The model under review builds one solid part; all positions refer to its coordinate system, in mm. Round coordinates to 2 decimals unless told otherwise and drop trailing zeros. Order: outer loops, then holes, each group sorted by start corner. A loop starts at its lowest first (then second) coordinate and runs counter-clockwise, first axis right, second up. Notation, with made-up numbers: M 27.5,-28.5 L 43.5,-28.5 A8 ccw 43.5,-20.5 Z; hole C -15.75,-3 d7. An arc over 180 degrees is marked long. One line per item, written item: value. Start each with the question number.
from build123d import *

# Parameters (mm, degrees)
SKETCH_1_W                   = 80
SKETCH_1_H                   = 50
EXTRUDE_1_DEPTH              = 3
EXTRUDE_2_DEPTH              = 3
SKETCH_8_R                   = 1.5
CUT_EXTRUDE_4_DEPTH          = 3
CUT_EXTRUDE_START            = -4
CUT_EXTRUDE_6_DEPTH          = 5
HOLE_WIZARD_M3_1_D           = 3
HOLE_WIZARD_M3_1_CSINK_D     = 6
HOLE_WIZARD_M3_1_CSINK_ANGLE = 90
MIRROR_7_COPY_1_DEPTH        = 3
MIRROR_START                 = -4
MIRROR_7_COPY_2_DEPTH        = 5
MIRROR_7_COPY_3_D            = 3
MIRROR_7_COPY_3_CSINK_D      = 6
MIRROR_7_COPY_3_CSINK_ANGLE  = 90
SKETCH_14_R                  = 10.1
CUT_EXTRUDE_7_DEPTH          = 4
SKETCH_15_R                  = 1.5
CUT_EXTRUDE_8_DEPTH          = 10
MIRROR_9_COPY_1_SKETCH_R     = 1.5
MIRROR_9_COPY_1_DEPTH        = 10


with BuildPart() as part:
    # 草图1 → 凸台-拉伸1 (new body)
    with BuildSketch(Plane(origin=(0, 0, 0), x_dir=(1, 0, 0), z_dir=(0, 1, 0))):
        Polygon((-15, -105.5), (-40, -25), (40, -25), (15, -105.5), align=None)
        Rectangle(SKETCH_1_W, SKETCH_1_H)
        Polygon((-15, 105.5), (15, 105.5), (40, 25), (-40, 25), align=None)
    extrude(amount=EXTRUDE_1_DEPTH)

    # 草图7 → 凸台-拉伸2 (add)
    with BuildSketch(Plane(origin=(0, 3, 0), x_dir=(1, 0, 0), z_dir=(0, 1, 0))):
        Polygon((15, 105.5), (25.392304845, 111.5), (31.392304845, 111.5), (34.279056191, 106.5), (31.392304845, 101.5), (27.5, 65.25), align=None)
    extrude_2 = extrude(amount=-EXTRUDE_2_DEPTH)

    # 草图8 → 切除-拉伸4 (cut)
    with BuildSketch(Plane(origin=(0, 3, 0), x_dir=(1, 0, 0), z_dir=(0, 1, 0))):
        with Locations((27, 106.5)):
            Circle(SKETCH_8_R)
    extrude(amount=-CUT_EXTRUDE_4_DEPTH, mode=Mode.SUBTRACT)

    # 草图9 → 切除-拉伸6 (cut)
    with BuildSketch(Plane(origin=(0, 3, 0), x_dir=(1, 0, 0), z_dir=(0, 1, 0)).offset(CUT_EXTRUDE_START)):
        Polygon((22.528576043, 65.783801312), (26.420880888, 102.033801312), (23.243297221, 103.222190391), (21.66924243, 105.948533263), (16.658152368, 102.627995852), (19.093364206, 84.205898582), (21.528576043, 65.783801312), align=None)
        Polygon((10.313400805, 97.671116845), (19.093364206, 84.205898582), (16.658152368, 102.627995852), (9.970725358, 98.196654308), align=None)
    cut_extrude_6 = extrude(amount=CUT_EXTRUDE_6_DEPTH, mode=Mode.SUBTRACT)

    # M3 六角凹锥坑螺钉的锥形沉头孔1 (through all)
    with Locations(Plane(origin=(0, 3, 0), x_dir=(1, 0, 0), z_dir=(0, 1, 0))):
        with Locations((27, 106.5), (32, 0)):
            hole_wizard_m3_1 = CounterSinkHole(HOLE_WIZARD_M3_1_D / 2, HOLE_WIZARD_M3_1_CSINK_D / 2, counter_sink_angle=HOLE_WIZARD_M3_1_CSINK_ANGLE)

    # 镜向5: M3 六角凹锥坑螺钉的锥形沉头孔1 across plane
    add(hole_wizard_m3_1.mirror(Plane(origin=(0, 0, 0), x_dir=(0, 0, 1), z_dir=(1, 0, 0))), mode=Mode.SUBTRACT)

    # 镜向6: 凸台-拉伸2, 切除-拉伸6, M3 六角凹锥坑螺钉的锥形沉头孔1 across plane
    add(extrude_2.mirror(Plane(origin=(0, 0, 0), x_dir=(0, 0, 1), z_dir=(1, 0, 0))))
    add(cut_extrude_6.mirror(Plane(origin=(0, 0, 0), x_dir=(0, 0, 1), z_dir=(1, 0, 0))), mode=Mode.SUBTRACT)
    add(hole_wizard_m3_1.mirror(Plane(origin=(0, 0, 0), x_dir=(0, 0, 1), z_dir=(1, 0, 0))), mode=Mode.SUBTRACT)

    # 镜向7: 凸台-拉伸2, 切除-拉伸6, M3 六角凹锥坑螺钉的锥形沉头孔1 across plane
    add(extrude_2.mirror(Plane.XY))
    add(cut_extrude_6.mirror(Plane.XY), mode=Mode.SUBTRACT)
    add(hole_wizard_m3_1.mirror(Plane.XY), mode=Mode.SUBTRACT)

    # 镜向7 copy 1 sketch → 镜向7 copy 1 (add)
    with BuildSketch(Plane(origin=(0, 3, 0), x_dir=(-1, 0, 0), z_dir=(0, 1, 0))):
        Polygon((15, 105.5), (25.392304845, 111.5), (31.392304845, 111.5), (34.279056191, 106.5), (31.392304845, 101.5), (27.5, 65.25), align=None)
    extrude(amount=-MIRROR_7_COPY_1_DEPTH)

    # 镜向7 copy 2 sketch → 镜向7 copy 2 (cut)
    with BuildSketch(Plane(origin=(0, 3, 0), x_dir=(-1, 0, 0), z_dir=(0, 1, 0)).offset(MIRROR_START)):
        Polygon((22.528576043, 65.783801312), (26.420880888, 102.033801312), (23.243297221, 103.222190391), (21.66924243, 105.948533263), (16.658152368, 102.627995852), (19.093364206, 84.205898582), (21.528576043, 65.783801312), align=None)
        Polygon((10.313400805, 97.671116845), (19.093364206, 84.205898582), (16.658152368, 102.627995852), (9.970725358, 98.196654308), align=None)
    extrude(amount=MIRROR_7_COPY_2_DEPTH, mode=Mode.SUBTRACT)

    # 镜向7 copy 3 (through all)
    with Locations(Plane(origin=(0, 3, 0), x_dir=(-1, 0, 0), z_dir=(0, 1, 0))):
        with Locations((27, 106.5), (32, 0)):
            CounterSinkHole(MIRROR_7_COPY_3_D / 2, MIRROR_7_COPY_3_CSINK_D / 2, counter_sink_angle=MIRROR_7_COPY_3_CSINK_ANGLE)

    # 草图14 → 切除-拉伸7 (cut, through all)
    with BuildSketch(Plane(origin=(0, 3, 0), x_dir=(1, 0, 0), z_dir=(0, 1, 0))):
        Circle(SKETCH_14_R)
        with Locations((0, -50)):
            Circle(SKETCH_14_R)
        with Locations((0, 50)):
            Circle(SKETCH_14_R)
    extrude(amount=-CUT_EXTRUDE_7_DEPTH, mode=Mode.SUBTRACT)

    # 草图15 → 切除-拉伸8 (cut)
    with BuildSketch(Plane.XZ):
        with Locations((-32, 15)):
            Circle(SKETCH_15_R)
        with Locations((-32, 30)):
            Circle(SKETCH_15_R)
        with Locations((-12, 65)):
            Circle(SKETCH_15_R)
        with Locations((-12, 30)):
            Circle(SKETCH_15_R)
    cut_extrude_8 = extrude(amount=-CUT_EXTRUDE_8_DEPTH, mode=Mode.SUBTRACT)

    # 镜向8: 切除-拉伸8 across plane
    add(cut_extrude_8.mirror(Plane(origin=(0, 0, 0), x_dir=(0, 0, 1), z_dir=(1, 0, 0))), mode=Mode.SUBTRACT)

    # 镜向9: 切除-拉伸8 across plane
    add(cut_extrude_8.mirror(Plane.XY), mode=Mode.SUBTRACT)

    # 镜向9 copy 1 sketch → 镜向9 copy 1 (cut)
    with BuildSketch(Plane(origin=(0, 0, 0), x_dir=(-1, 0, 0), z_dir=(0, -1, 0))):
        with Locations((-32, 15)):
            Circle(MIRROR_9_COPY_1_SKETCH_R)
        with Locations((-32, 30)):
            Circle(MIRROR_9_COPY_1_SKETCH_R)
        with Locations((-12, 65)):
            Circle(MIRROR_9_COPY_1_SKETCH_R)
        with Locations((-12, 30)):
            Circle(MIRROR_9_COPY_1_SKETCH_R)
    extrude(amount=-MIRROR_9_COPY_1_DEPTH, mode=Mode.SUBTRACT)


solid = part.part
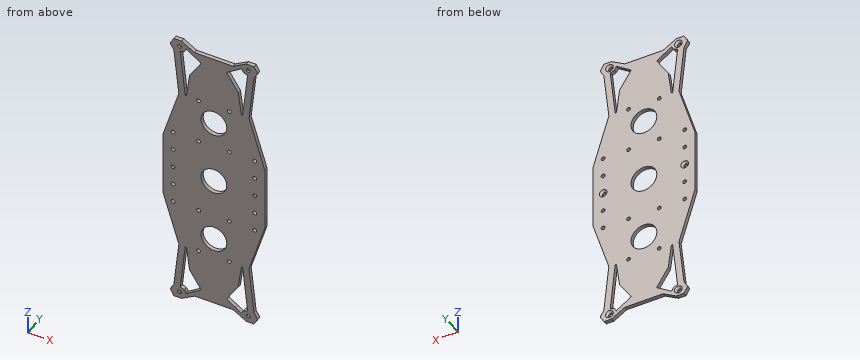
Item 1: Clearance check with flat-ended pins moving along their axes: P1, Ø1, axis at y = 1.5, z = 72.5, coming from the -X side; P2, Ø12, axis at x = 0, z = -50, coming from the +Y side; P3, Ø1.5, axis at x = 3, y = 1.5, coming from the +Z side; P4, Ø5, axis at x = 27, z = 106.5, coming from the +Y side. State where each tip first meets the part, or that it passes through.
Item 2: Consider section B-B, the plane y = 2.35. Count the separate pieces of the cut face and the enclosed holes in it, then the cut area to 3 significant figures.
Item 3: Consider section C-C, the plane z = 50. Give the boundary of the cut face in (x, y), then the cut area to 3 significant figures.
Item 4: Consider section A-A, the plane z = 87. Give the boundary of the cut face in (x, y), then the cut area to 3 significant figures.
Item 5: Wall thickness on L1, parallel to Z at x = 0, y = 2.35; L2, parallel to X at y = 0.8, z = -106.5; L3, parallel to X at y = 1.7, z = -14.5: over which ranges is each line inside the solid? List them lowest first.
Item 6: Consider section D-D, the plane z = -93.5. Give the boundary of the cut face in (x, y), then the cut area to 3 significant figures.
Computed:
1. P1: stops at x = -28.33
1. P2: passes through
1. P3: stops at z = 105.5
1. P4: stops at y = 2.5
2. separate pieces: 1
2. enclosed holes: 29
2. area: 12,200 mm^2
3. outline: M -32.24,0 L -10.1,0 L -10.1,3 L -32.24,3 Z; M 10.1,0 L 32.24,0 L 32.24,3 L 10.1,3 Z
3. area: 133 mm^2
4. outline: M -29.84,0 L -24.81,0 L -24.81,3 L -29.84,3 Z; M -17.27,0 L 17.27,0 L 17.27,3 L -17.27,3 Z; M 24.81,0 L 29.84,0 L 29.84,3 L 24.81,3 Z
4. area: 134 mm^2
5. L1: z = -105.5 to -60.1, -39.9 to -10.1, 10.1 to 39.9, 60.1 to 105.5
5. L2: x = -34.28 to -28.5, -25.5 to -16.73, 16.73 to 25.5, 28.5 to 34.28
5. L3: x = -40 to -33.41, -30.59 to 30.59, 33.41 to 40
6. outline: M -30.53,0 L -25.5,0 L -25.5,3 L -30.53,3 Z; M -13.03,0 L 13.03,0 L 13.03,3 L -13.03,3 Z; M 25.5,0 L 30.53,0 L 30.53,3 L 25.5,3 Z
6. area: 108 mm^2
